```python
from build123d import *

# Parameters (mm, degrees)
BOSS_EXTRUDE1_DEPTH = 22.225
SKETCH2_R           = 6.35
CUT_EXTRUDE1_DEPTH  = 3.175
SKETCH3_R           = 2.54
CUT_EXTRUDE2_DEPTH  = 3.175


with BuildPart() as part:
    # Sketch1 → Boss-Extrude1 (new body)
    with BuildSketch(Plane(origin=(0, 0, 0), x_dir=(1, 0, 0), z_dir=(0, 1, 0))):
        Polygon((22.225, 14.2875), (22.225, -17.4625), (25.4, -17.4625), (25.4, 17.4625), (-25.4, 17.4625), (-25.4, 14.2875), align=None)
    extrude(amount=BOSS_EXTRUDE1_DEPTH)

    # Sketch2 → Cut-Extrude1 (cut)
    with BuildSketch(Plane(origin=(25.4, 0, 0), x_dir=(0, 0, -1), z_dir=(1, 0, 0))):
        with Locations((-4.7625, 12.7)):
            Circle(SKETCH2_R)
    extrude(amount=-CUT_EXTRUDE1_DEPTH, mode=Mode.SUBTRACT)

    # Sketch3 → Cut-Extrude2 (cut)
    with BuildSketch(Plane.XY.offset(-14.2875)):
        with Locations((-12.7, 12.7)):
            Circle(SKETCH3_R)
        with Locations((0, 12.7)):
            Circle(SKETCH3_R)
        with Locations((12.7, 12.7)):
            Circle(SKETCH3_R)
    extrude(amount=-CUT_EXTRUDE2_DEPTH, mode=Mode.SUBTRACT)


solid = part.part
```
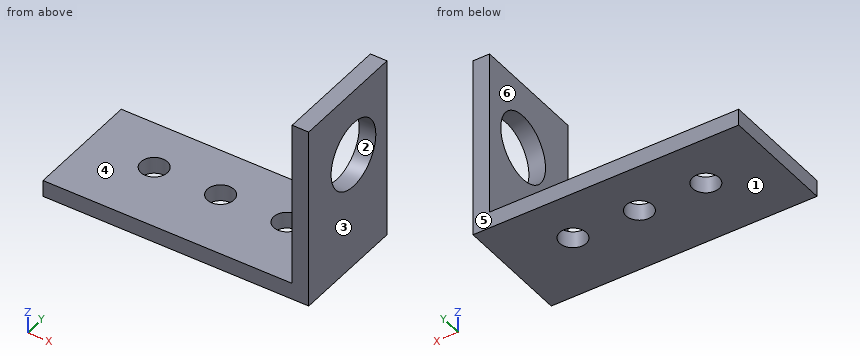
Model file for the job. Use its own axes, mm. Face numbers are marked on the shaded views. A direction names the side the tool comes from. Round coordinates to 2 decimals unless told otherwise and drop trailing zeros. Order: outer loops, then holes, each group sorted by start corner. A loop starts at its lowest first (then second) coordinate and runs counter-clockwise, first axis right, second up. Notation, with made-up numbers: M -2,-5.5 L 40,-5.5 A9 cw 40,6.5 Z; hole C 32.25,-30 d10. An arc over 180 degrees is marked long. Use CSV: the item, a comma, the result in double quotes.
Item 1: Saw through at B-B (y = 9.25). List the corners of the cut face in (x, z) (1 decimal), plus the area to 3 significant figures.
Worked answers:
outline,"M -25.4,-17.5 L 25.4,-17.5 L 25.4,-0.6 L 22.2,-0.6 L 22.2,-14.3 L -25.4,-14.3 Z; M 22.2,10.1 L 25.4,10.1 L 25.4,17.5 L 22.2,17.5 Z"
area,"228 mm²"
Item 2: Pull direction Z, two halves, no side cores. Call the marked faces 1, 2, 3 and 4: released by +Z, released by -Z, zero draft, split by the parting line, or undercut.
Worked answers:
face 1,"released by -Z"
face 2,"undercut"
face 3,"zero draft"
face 4,"released by +Z"
Item 3: Saw through at D-D (y = 14.5). List the corners of the cut face in (x, z) (1 decimal), plus the area to 3 significant figures.
Worked answers:
outline,"M -25.4,-17.5 L -14.5,-17.5 L -14.5,-14.3 L -25.4,-14.3 Z; M -10.9,-17.5 L -1.8,-17.5 L -1.8,-14.3 L -10.9,-14.3 Z; M 1.8,-17.5 L 10.9,-17.5 L 10.9,-14.3 L 1.8,-14.3 Z; M 14.5,-17.5 L 25.4,-17.5 L 25.4,-1.3 L 22.2,-1.3 L 22.2,-14.3 L 14.5,-14.3 Z; M 22.2,10.9 L 25.4,10.9 L 25.4,17.5 L 22.2,17.5 Z"
area,"189 mm²"
Item 4: Which spindle directions (+Z, -Z, +X, -X, +Y, -Y) get a long thin tool onto all of the face, cutting with end or side? Do the marked faces 5 and 6. Say none if no direction does.
Worked answers:
face 5,"+Z, -Z, +X, -X, +Y"
face 6,"+Z, -X, +Y, -Y"
Item 5: Probe probe 1 along Y at (x, z) = (-12.7, -15.4) (3 decimals); probe 2 along Z at (x, y) = (-9.5, 17); probe 3 along X at (y, z) = (4.75, -9.5) (3 decimals). List the from-to ranges inside material, lowest first.
Worked answers:
probe 1,"0 to 10.16, 15.24 to 22.225"
probe 2,"-17.46 to -14.29"
probe 3,"22.225 to 25.4"
Item 6: Pin check, flat tips, straight feed: pin 1 (4 mm diameter, centred on y = 5, z = 2.5, fed in from -X) (3 decimals); pin 2 (8 mm diameter, centred on x = -12.7, y = 12.7, fed in from +Z). Stop position of each tip, or through.
Worked answers:
pin 1,"x = 22.225"
pin 2,"z = -14.29"
Item 7: Saw through at C-C (z = 3.5). List the corners of the cut face in (x, y) (3 decimals), plus the area to 3 significant figures.
Worked answers:
outline,"M 22.225,0 L 25.4,0 L 25.4,6.477 L 22.225,6.477 Z; M 22.225,18.923 L 25.4,18.923 L 25.4,22.225 L 22.225,22.225 Z"
area,"31.0 mm²"
Item 8: Saw through at A-A (x = 0). List the corners of the cut face in (y, z) (1 decimal).
Worked answers:
outline,"M 0,-17.5 L 10.2,-17.5 L 10.2,-14.3 L 0,-14.3 Z; M 15.2,-17.5 L 22.2,-17.5 L 22.2,-14.3 L 15.2,-14.3 Z"
